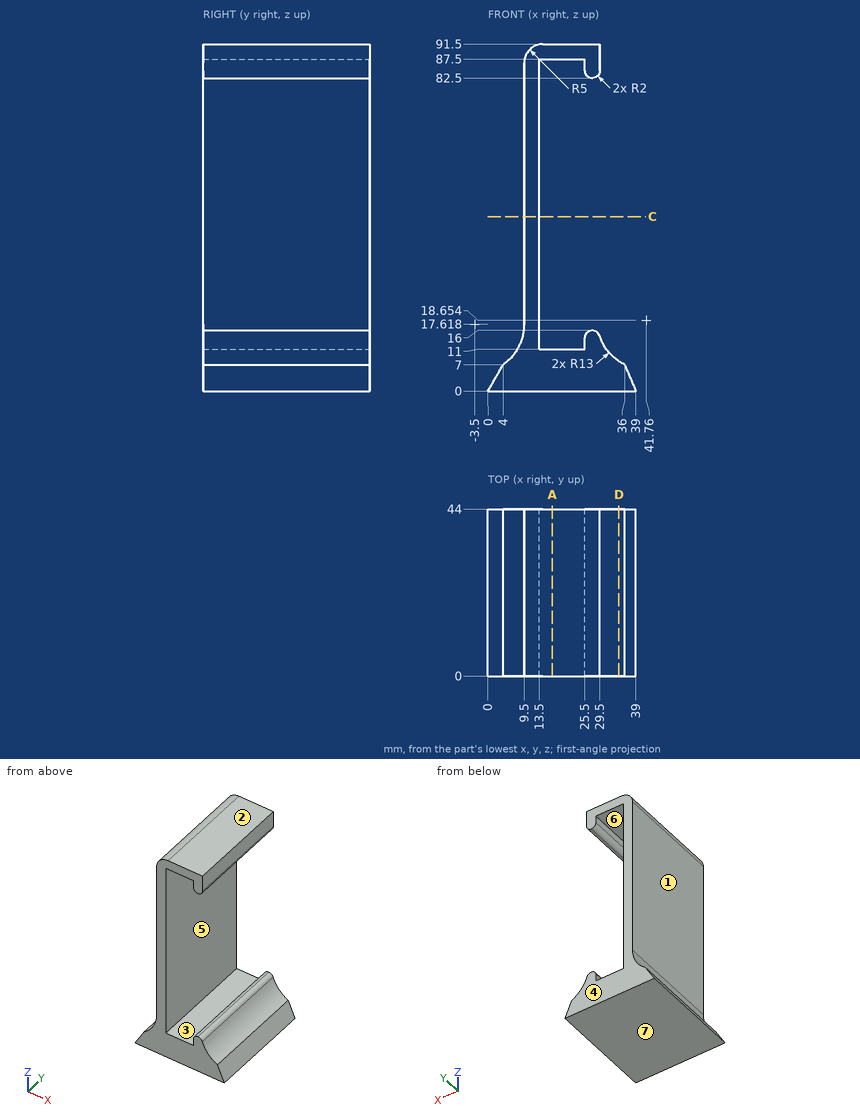
Input: dimensioned drawing with shaded views. Units: mm. Origin: part minimum x, y, z. A direction names the side the tool comes from. Give positions to 0.01 mm unless a question says otherwise; leave off trailing zeros. Write each loop counter-clockwise with the first axis right and the second up, starting at its lowest first coordinate (ties: lowest second). Pieces come first, ordered by that corner, then holes. Notation, with made-up numbers: M 57.25,-27.5 L 78.25,-27.5 A28 cw 78.25,11.5 Z; hole C -6,25.25 d2. An arc over 180 degrees is marked long. Write item = value, one per line. Start each with the question number.
1) Cut plane C-C on z = 46. Return the cut outline in (x, y).
2) Reachability of the marked faces 1, 2 and 3 from +Z, -Z, +X, -X, +Y, -Y: full face, straight path, thin tool, end or side. Return the list, or none.
3) First-contact query: pin 1 Ø3.5 at (y, z) = (24, 13) entering from -X; pin 2 Ø22 at (y, z) = (13.5, 56) entering from +X; pin 3 Ø1.5 at (y, z) = (7, 13.5) entering from +X. Flat tips, straight axial feed; report the tip coordinate or a pass-through.
4) Material intervals for line 1 along Z through (x, y) = (22.5, 35.5); line 2 along X through (y, z) = (34, 60); line 3 along X through (y, z) = (3, 14) (1 decimal), sorted ascending. Write a range as [from, to].
5) Draft query along Z for the marked faces 4, 5, 6 and 7. Return one class per face: +Z half, -Z half, draft (parallel to the pull), parting line (faces both ways), or undercut.
6) Cut plane A-A on x = 17. Return the cut outline in (y, z).
7) Cut plane D-D on x = 34.5. Return the cut outline in (y, z).
Solved:
q1.outline = M 9.5,0 L 13.5,0 L 13.5,44 L 9.5,44 Z
q2.face_1 = +Z, -X, +Y, -Y
q2.face_2 = +Z, +X, -X, +Y, -Y
q2.face_3 = +Y, -Y
q3.pin_1 = 7.83
q3.pin_2 = 13.5
q3.pin_3 = 30.18
q4.line_1 = [0, 11], [87.5, 91.5]
q4.line_2 = [9.5, 13.5]
q4.line_3 = [9, 13.5], [25.5, 29.6]
q5.face_4 = draft
q5.face_5 = undercut
q5.face_6 = undercut
q5.face_7 = -Z half
q6.outline = M 0,0 L 44,0 L 44,11 L 0,11 Z; M 0,87.5 L 44,87.5 L 44,91.5 L 0,91.5 Z
q7.outline = M 0,0 L 44,0 L 44,7.87 L 0,7.87 Z
